For this review, take the finished solid that the model builds, in its own axes (mm). Coordinates: 2 decimals unless noted, no trailing zeros. Loops run counter-clockwise (first coordinate to the right, second up) from the corner with the lowest first, then second, coordinate; pieces in that order, holes last.
1. Take a section at D-D, the plane z = -0.35. State the section outline as (x, y) points.
2. Clearance check with a flat-ended pin moving along its axis: P1, Ø9, axis at x = -35.79, y = -62.35, coming from the -Z side. State where the tip first meets the part, or that it passes through.
3. Take a section at A-A, the plane x = -70.5. State the section outline as (y, z) points, then the cut area to 3 significant figures.
4. Take a section at C-C, the plane y = -61.25. State the section outline as (x, z) points, then the cut area to 3 significant figures.
5. To check wall thickness, follow probe 1 along Y at (x, z) = (-69, -0.55); probe 2 along X at (y, z) = (-62.25, -0.5); probe 3 along X at (y, z) = (-59.75, -0.3). State the ranges of each line that lie inside material, in increasing order.
6. Take a section at B-B, the plane y = -68.25. State the section outline as (x, z) points.
```python
from build123d import *

# Parameters (mm, degrees)
SKETCH1_W               = 44
SKETCH1_H               = 18
BOSS_EXTRUDE1_DEPTH     = 2
CUT_EXTRUDE3_DEPTH      = 1
CUT_EXTRUDE3_DEPTH_BACK = 2
SKETCH8_R               = 3.5
CUT_EXTRUDE4_DEPTH      = 2.8
SKETCH9_R               = 3.5
CUT_EXTRUDE5_DEPTH      = 2.8


with BuildPart() as part:
    # Sketch1 → Boss-Extrude1 (new body)
    with BuildSketch(Plane.XY):
        with Locations((-52.289658906, -63.346772489)):
            Rectangle(SKETCH1_W, SKETCH1_H)
    extrude(amount=-BOSS_EXTRUDE1_DEPTH)

    # Sketch7 → Cut-Extrude3 (cut, two sides)
    with BuildSketch(Plane.XY) as cut_extrude3_sk:
        with BuildLine():
            Line((-45.289658906, -150.610965153), (-45.289658906, -72.346772489))
            ThreePointArc((-45.289658906, -72.346772489), (-52.289658906, -65.346772489), (-59.289658906, -72.346772489))
            Line((-59.289658906, -72.346772489), (-59.289658906, -150.610965153))
            Line((-59.289658906, -150.610965153), (-59.289658906, -307.13935048))
            Line((-59.289658906, -307.13935048), (-45.289658906, -307.13935048))
            Line((-45.289658906, -307.13935048), (-45.289658906, -150.610965153))
        make_face()
    extrude(amount=CUT_EXTRUDE3_DEPTH, mode=Mode.SUBTRACT)
    extrude(cut_extrude3_sk.sketch, amount=-CUT_EXTRUDE3_DEPTH_BACK, mode=Mode.SUBTRACT)

    # Sketch8 → Cut-Extrude4 (cut)
    with BuildSketch(Plane.XY):
        with Locations((-68.789658906, -62.346772489)):
            Circle(SKETCH8_R)
    extrude(amount=-CUT_EXTRUDE4_DEPTH, mode=Mode.SUBTRACT)

    # Sketch9 → Cut-Extrude5 (cut)
    with BuildSketch(Plane.XY):
        with Locations((-35.789658906, -62.346772489)):
            Circle(SKETCH9_R)
    extrude(amount=-CUT_EXTRUDE5_DEPTH, mode=Mode.SUBTRACT)


solid = part.part
```
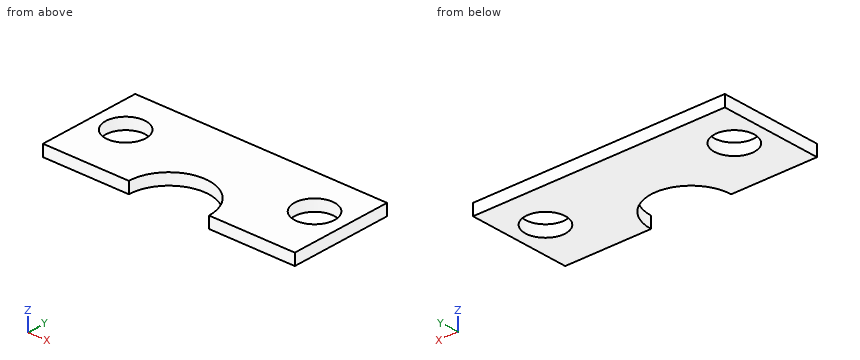
Results list:
1. outline: (-74.29, -72.35) - (-59.29, -72.35) arc R7 cw to (-45.29, -72.35) - (-30.29, -72.35) - (-30.29, -54.35) - (-74.29, -54.35) - close; hole circle Ø7 at (-68.79, -62.35); hole circle Ø7 at (-35.79, -62.35)
2. P1: stops at z = -2
3. outline: (-72.35, -2) - (-65.4, -2) - (-65.4, 0) - (-72.35, 0) - close; (-59.29, -2) - (-54.35, -2) - (-54.35, 0) - (-59.29, 0) - close
3. area: 23.8 mm2
4. outline: (-74.29, -2) - (-72.11, -2) - (-72.11, 0) - (-74.29, 0) - close; (-65.47, -2) - (-39.11, -2) - (-39.11, 0) - (-65.47, 0) - close; (-32.47, -2) - (-30.29, -2) - (-30.29, 0) - (-32.47, 0) - close
4. area: 61.4 mm2
5. probe 1: y = -72.35 to -65.84, -58.85 to -54.35
5. probe 2: x = -74.29 to -72.29, -65.29 to -39.29, -32.29 to -30.29
5. probe 3: x = -74.29 to -71.14, -66.44 to -38.14, -33.44 to -30.29
6. outline: (-74.29, -2) - (-57.97, -2) - (-57.97, 0) - (-74.29, 0) - close; (-46.61, -2) - (-30.29, -2) - (-30.29, 0) - (-46.61, 0) - close
